Source: CAD feature listing. Evaluate the final solid. Frame: model axes, mm. Face numbers are marked on the shaded views. A direction names the side the tool comes from. Coordinates: 2 decimals unless noted, no trailing zeros. Order: outer loops, then holes, each group sorted by start corner. A loop starts at its lowest first (then second) coordinate and runs counter-clockwise, first axis right, second up.
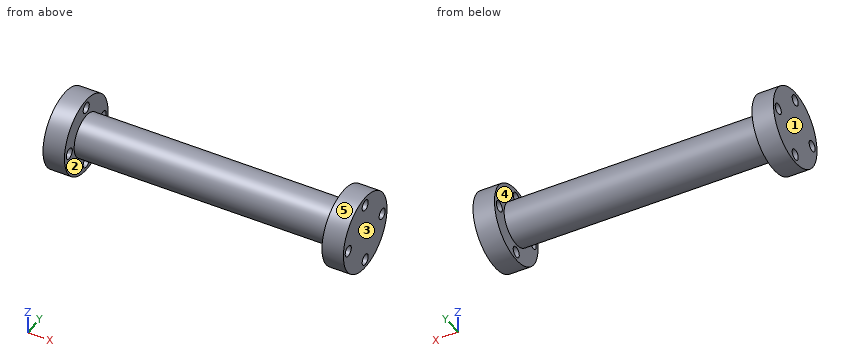
```python
from build123d import *

# Parameters (mm, degrees)
HOLE_WIZARD_M3_1_D     = 2.5
HOLE_WIZARD_M3_1_DEPTH = 5
HOLE_WIZARD_M3_1_TIP   = 0.751075774
HOLE_WIZARD_M3_2_D     = 2.5
HOLE_WIZARD_M3_2_DEPTH = 5
HOLE_WIZARD_M3_2_TIP   = 0.751075774


with BuildPart() as part:
    # 草图1 → 旋转1 (revolve)
    with BuildSketch(Plane.XY, mode=Mode.PRIVATE) as revolve_1_sk:
        Polygon((-43.905067628, 0), (26.094932372, 0), (26.094932372, 9), (21.094932372, 9), (21.094932372, 5), (-38.905067628, 5), (-38.905067628, 9), (-43.905067628, 9), align=None)
    revolve(revolve_1_sk.sketch.rotate(Axis((-43.905067628, 0, 0), (1, 0, 0)), 90), axis=Axis((-43.905067628, 0, 0), (1, 0, 0)))

    # M3 螺纹孔1
    with Locations(Plane.ZY.offset(43.905067628)):
        with Locations((7, 0), (0, 7), (-7, 0), (0, -7)):
            Hole(HOLE_WIZARD_M3_1_D / 2, depth=HOLE_WIZARD_M3_1_DEPTH)
            with Locations((0, 0, -(HOLE_WIZARD_M3_1_DEPTH + HOLE_WIZARD_M3_1_TIP / 2))):  # 118° drill point
                Cone(0, HOLE_WIZARD_M3_1_D / 2, HOLE_WIZARD_M3_1_TIP, mode=Mode.SUBTRACT)

    # M3 螺纹孔2
    with Locations(Plane(origin=(26.094932372, 0, 0), x_dir=(0, 0, -1), z_dir=(1, 0, 0))):
        with Locations((0, -7), (7, 0), (0, 7), (-7, 0)):
            Hole(HOLE_WIZARD_M3_2_D / 2, depth=HOLE_WIZARD_M3_2_DEPTH)
            with Locations((0, 0, -(HOLE_WIZARD_M3_2_DEPTH + HOLE_WIZARD_M3_2_TIP / 2))):  # 118° drill point
                Cone(0, HOLE_WIZARD_M3_2_D / 2, HOLE_WIZARD_M3_2_TIP, mode=Mode.SUBTRACT)


solid = part.part
```
1. Contact query for flat-ended pins moving along their axis: P1, Ø1.5, axis at x = 5.5, z = -3, coming from the -Y side; P2, Ø5, axis at x = -27, z = 6, coming from the +Y side; P3, Ø1, axis at x = -35, y = 2.5, coming from the +Z side; P4, Ø3, axis at y = 7, z = 0, coming from the -X side. Output: stop coordinate, or through.
2. Draft query along X for the marked faces 3, 4 and 5. Return one class per face: +X half, -X half, draft (parallel to the pull), parting line (faces both ways), or undercut.
3. Section query A-A, the plane z = 0. Output: boundary loops of the cut face in (x, y), plus the area to 3 significant figures.
4. Access query for the marked faces 1 and 2. Directions: +Z, -Z, +X, -X, +Y, -Y. A direction counts if a zero-diameter tool reaches every point of the face in a straight line with its end or side. Return the directions, or none.
5. Material intervals for line 1 along Y through (x, z) = (24.3, 0); line 2 along X through (y, z) = (-3.25, -7.5); line 3 along Y through (x, z) = (24.5, -7), sorted ascending.
6. Section query C-C, the plane z = 7.5. Output: boundary loops of the cut face in (x, y), plus the area to 3 significant figures.
7. Section query D-D, the plane y = -7. Output: boundary loops of the cut face in (x, z), plus the area to 3 significant figures.
Answer key:
1. P1: stops at y = -4.47
1. P2: stops at y = 3.57
1. P3: stops at z = 4.58
1. P4: stops at x = -43.91
2. face 3: +X half
2. face 4: undercut
2. face 5: draft
3. outline: (-43.91, -9) - (-38.91, -9) - (-38.91, -8.25) - (-43.91, -8.25) - close; (-43.91, -5.75) - (-38.91, -5.75) - (-38.91, -5) - (21.09, -5) - (21.09, -5.75) - (26.09, -5.75) - (26.09, 5.75) - (21.09, 5.75) - (21.09, 5) - (-38.91, 5) - (-38.91, 5.75) - (-43.91, 5.75) - close; (-43.91, 8.25) - (-38.91, 8.25) - (-38.91, 9) - (-43.91, 9) - close; (21.09, -9) - (26.09, -9) - (26.09, -8.25) - (21.09, -8.25) - close; (21.09, 8.25) - (26.09, 8.25) - (26.09, 9) - (21.09, 9) - close
3. area: 730 mm2
4. face 1: +Z, -Z, -X, +Y, -Y
4. face 2: none
5. line 1: y = -9 to -8.25, -5.75 to 5.75, 8.25 to 9
5. line 2: x = -43.91 to -38.91, 21.09 to 26.09
5. line 3: y = -5.66 to -1.25, 1.25 to 5.66
6. outline: (-43.91, -4.97) - (-38.91, -4.97) - (-38.91, -1.15) - (-43.91, -1.15) - close; (-43.91, 1.15) - (-38.91, 1.15) - (-38.91, 4.97) - (-43.91, 4.97) - close; (21.09, -4.97) - (26.09, -4.97) - (26.09, -1.15) - (21.09, -1.15) - close; (21.09, 1.15) - (26.09, 1.15) - (26.09, 4.97) - (21.09, 4.97) - close
6. area: 76.6 mm2
7. outline: (-43.91, -5.66) - (-38.91, -5.66) - (-38.91, -1.25) - (-43.91, -1.25) - close; (-43.91, 1.25) - (-38.91, 1.25) - (-38.91, 5.66) - (-43.91, 5.66) - close; (21.09, -5.66) - (26.09, -5.66) - (26.09, -1.25) - (21.09, -1.25) - close; (21.09, 1.25) - (26.09, 1.25) - (26.09, 5.66) - (21.09, 5.66) - close
7. area: 88.1 mm2
